The listing builds one solid part. Answer for the finished solid, in the listing's coordinates (mm). Face numbers are marked on the shaded views. A direction names the side the tool comes from. Round coordinates to 2 decimals unless told otherwise and drop trailing zeros. Order: outer loops, then holes, each group sorted by start corner. A loop starts at its lowest first (then second) coordinate and runs counter-clockwise, first axis right, second up. Notation, with made-up numbers: (25.5, 89) -> (68.5, 89) arc R10 cw to (68.5, 97) -> close; hole circle Ø2 at (-20, 73.25). An arc over 180 degrees is marked (long way). Return JSON: item names as keys, results as strings. Group by question number.
(1) The part is cut by section D-D (y = 15). Determine the outline of the cut face in (x, z), plus the area to 3 significant figures.
(2) The part is cut by section B-B (y = 7). Count the separate pieces of the cut face and the enclosed holes in it, plus the area to 3 significant figures.
(3) The part is cut by section A-A (z = 47). Determine the outline of the cut face in (x, y).
(4) Consider line 1 (Z direction, x = 54.5, y = 6); line 2 (X direction, y = 4, z = 47); line 3 (X direction, y = 14, z = -4.5). Determine where each line is inside the solid, lowest interval first. Write a range as [from, to].
(5) The part is cut by section C-C (x = 0). Determine the outline of the cut face in (y, z), plus the area to 3 significant figures.
(6) Which of the six approach directions +Z, -Z, +X, -X, +Y, -Y give full straight-line access (tool end or side, diameter ignored) to the marked faces 5, 6, 7 and 8?
(7) Determine the mould class of the marked faces 1, 2, 3 and 4 for opening direction Z: +Z half, -Z half, draft (parallel to the pull), parting line (faces both ways), or undercut.
(8) Each of these flat-tipped pins is pushed along its axis until it touches: pin 1 (1.5 mm diameter, centred on x = 1, y = 17.5, fed in from +Z); pin 2 (6.5 mm diameter, centred on y = 9, z = 18.5, fed in from +X); pin 3 (12 mm diameter, centred on y = 25.5, z = 17, fed in from -X). Where does it stop, or does it pass through?
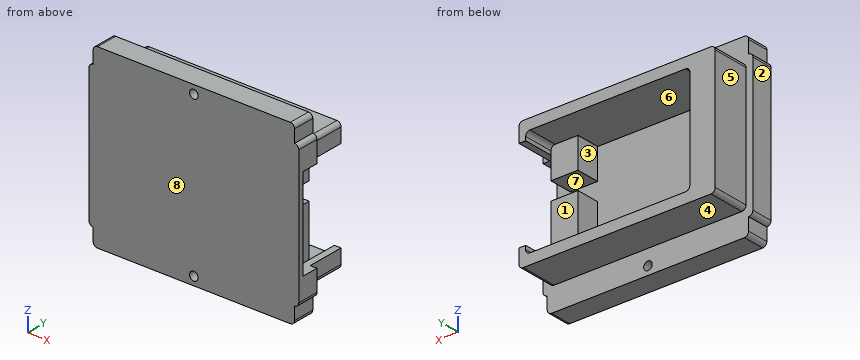
from build123d import *

# Parameters (mm, degrees)
SKETCH1_W           = 124
SKETCH1_H           = 84
BOSS_EXTRUDE1_DEPTH = 35
SKETCH2_W           = 97
SKETCH2_H           = 63.5
CUT_EXTRUDE1_DEPTH  = 32
SKETCH4_W           = 8
SKETCH4_H           = 54
CUT_EXTRUDE2_DEPTH  = 32
FILLET2_R           = 2.5
CUT_EXTRUDE3_DEPTH  = 22
FILLET4_R           = 2.5
SKETCH9_W           = 119
SKETCH9_H           = 13
BOSS_EXTRUDE3_DEPTH = 10
SKETCH11_W          = 119
SKETCH11_H          = 13
BOSS_EXTRUDE4_DEPTH = 10
SKETCH12_R          = 2.5
CUT_EXTRUDE6_DEPTH  = 84.857021173
FILLET5_R           = 2.5
BOSS_EXTRUDE5_DEPTH = 14


with BuildPart() as part:
    # Sketch1 → Boss-Extrude1 (new body)
    with BuildSketch(Plane(origin=(0, 0, 0), x_dir=(1, 0, 0), z_dir=(0, 1, 0))):
        Rectangle(SKETCH1_W, SKETCH1_H)
    extrude(amount=BOSS_EXTRUDE1_DEPTH)

    # Sketch2 → Cut-Extrude1 (cut)
    with BuildSketch(Plane(origin=(0, 35, 0), x_dir=(1, 0, 0), z_dir=(0, 1, 0))):
        with Locations((5.5, 0)):
            Rectangle(SKETCH2_W, SKETCH2_H)
    extrude(amount=-CUT_EXTRUDE1_DEPTH, mode=Mode.SUBTRACT)

    # Sketch4 → Cut-Extrude2 (cut)
    with BuildSketch(Plane(origin=(0, 35, 0), x_dir=(1, 0, 0), z_dir=(0, 1, 0))):
        with Locations((58, 0)):
            Rectangle(SKETCH4_W, SKETCH4_H)
    extrude(amount=-CUT_EXTRUDE2_DEPTH, mode=Mode.SUBTRACT)

    # Fillet2
    fillet2_edges = [part.edges().sort_by_distance(p)[0] for p in [
        (-43, 19, 31.75),
        (-43, 19, -31.75),
        (54, 19, -31.75),
        (54, 19, 31.75),
    ]]
    fillet(fillet2_edges, radius=FILLET2_R)

    # Sketch6 → Cut-Extrude3 (cut)
    with BuildSketch(Plane(origin=(0, 35, 0), x_dir=(1, 0, 0), z_dir=(0, 1, 0))):
        Polygon((-62, 42), (62, 42), (62, 27), (58, 27), (58, 38), (-58, 38), (-58, -38), (58, -38), (58, -27), (62, -27), (62, -42), (-62, -42), align=None)
    extrude(amount=-CUT_EXTRUDE3_DEPTH, mode=Mode.SUBTRACT)

    # Fillet4
    fillet4_edges = [part.edges().sort_by_distance(p)[0] for p in [
        (62, 6.5, 42),
        (-62, 6.5, 42),
        (-62, 6.5, -42),
        (62, 6.5, -42),
        (58, 24, -38),
        (-58, 24, -38),
        (-58, 24, 38),
        (58, 24, 38),
    ]]
    fillet(fillet4_edges, radius=FILLET4_R)

    # Sketch9 → Boss-Extrude3 (add)
    with BuildSketch(Plane(origin=(0, 0, -42), x_dir=(-1, 0, 0), z_dir=(0, 0, -1))):
        with Locations((0, 6.5)):
            Rectangle(SKETCH9_W, SKETCH9_H)
    extrude(amount=BOSS_EXTRUDE3_DEPTH)

    # Sketch11 → Boss-Extrude4 (add)
    with BuildSketch(Plane.XY.offset(42)):
        with Locations((0, 6.5)):
            Rectangle(SKETCH11_W, SKETCH11_H)
    extrude(amount=BOSS_EXTRUDE4_DEPTH)

    # Sketch12 → Cut-Extrude6 (cut, through all)
    with BuildSketch(Plane(origin=(0, 13, 0), x_dir=(1, 0, 0), z_dir=(0, 1, 0))):
        with Locations(Location((0, 47, 0), (0, 0, 270))):
            Circle(SKETCH12_R)
        with Locations(Location((0, -47, 0), (0, 0, 270))):
            Circle(SKETCH12_R)
    extrude(amount=-CUT_EXTRUDE6_DEPTH, mode=Mode.SUBTRACT)

    # Fillet5
    fillet5_edges = [part.edges().sort_by_distance(p)[0] for p in [
        (59.5, 6.5, -52),
        (-59.5, 6.5, -52),
        (-59.5, 6.5, 52),
        (59.5, 6.5, 52),
    ]]
    fillet(fillet5_edges, radius=FILLET5_R)

    # Sketch13 → Boss-Extrude5 (add)
    with BuildSketch(Plane(origin=(0, 3, 0), x_dir=(1, 0, 0), z_dir=(0, 1, 0))):
        with BuildLine():
            Line((38, 31.75), (38, -3.25))
            Line((38, -3.25), (54, -3.25))
            Line((54, -3.25), (54, 27))
            Line((54, 27), (54, 29.25))
            ThreePointArc((54, 29.25), (53.267766953, 31.017766953), (51.5, 31.75))
            Line((51.5, 31.75), (38, 31.75))
        make_face()
        with BuildLine():
            Line((38, -31.75), (38, -13.75))
            Line((38, -13.75), (54, -13.75))
            Line((54, -13.75), (54, -27))
            Line((54, -27), (54, -29.25))
            ThreePointArc((54, -29.25), (53.267766953, -31.017766953), (51.5, -31.75))
            Line((51.5, -31.75), (38, -31.75))
        make_face()
    extrude(amount=BOSS_EXTRUDE5_DEPTH)


solid = part.part
Answer below:
{
 "1": {"outline": "(-58, -35.5) arc R2.5 ccw to (-55.5, -38) -> (55.5, -38) arc R2.5 ccw to (58, -35.5) -> (58, -27) -> (54, -27) -> (54, 3.25) -> (38, 3.25) -> (38, -31.75) -> (-40.5, -31.75) arc R2.5 cw to (-43, -29.25) -> (-43, 29.25) arc R2.5 cw to (-40.5, 31.75) -> (38, 31.75) -> (38, 13.75) -> (54, 13.75) -> (54, 27) -> (58, 27) -> (58, 35.5) arc R2.5 ccw to (55.5, 38) -> (-55.5, 38) arc R2.5 ccw to (-58, 35.5) -> close", "area": "3,290 mm²"},
 "2": {"separate pieces": "1", "enclosed holes": "2", "area": "7,010 mm²"},
 "3": {"outline": "(-59.5, 0) -> (-2.5, 0) -> (-2.5, 13) -> (-59.5, 13) -> close; (2.5, 0) -> (59.5, 0) -> (59.5, 13) -> (2.5, 13) -> close"},
 "4": {"line 1": "z = [-52, -27], [27, 52]", "line 2": "x = [-59.5, -2.5], [2.5, 59.5]", "line 3": "x = [-58, -43], [38, 54]"},
 "5": {"outline": "(0, -52) -> (13, -52) -> (13, -49.5) -> (0, -49.5) -> close; (0, -44.5) -> (13, -44.5) -> (13, -38) -> (35, -38) -> (35, -31.75) -> (3, -31.75) -> (3, 31.75) -> (35, 31.75) -> (35, 38) -> (13, 38) -> (13, 44.5) -> (0, 44.5) -> close; (0, 49.5) -> (13, 49.5) -> (13, 52) -> (0, 52) -> close", "area": "862 mm²"},
 "6": {"face 5": "+Z, -Z, -X, +Y", "face 6": "+Y", "face 7": "+X, +Y", "face 8": "+Z, -Z, +X, -X, -Y"},
 "7": {"face 1": "undercut", "face 2": "draft", "face 3": "undercut", "face 4": "-Z half"},
 "8": {"pin 1": "stops at z = 38", "pin 2": "stops at x = 54", "pin 3": "stops at x = -58"}
}
